```python
from build123d import *

# Parameters (mm, degrees)
ESQUISSE1_W             = 30
ESQUISSE1_H             = 1
ESQUISSE7_R             = 1.7
ENL_V_MAT_EXTRU_1_DEPTH = 33.023428923
ESQUISSE8_R             = 1.6
ENL_V_MAT_EXTRU_2_DEPTH = 32.705677725


with BuildPart() as part:
    # Balayage1: sweep along a path in Esquisse6
    with BuildLine(Plane(origin=(0, 0, 0), x_dir=(0, 0, -1), z_dir=(1, 0, 0))) as balayage1_path:
        Line((0, 0), (20, 0))
        Line((20, 0), (20, -20))
    # Esquisse1 → Balayage1 (sweep)
    with BuildSketch(Plane.XY):
        Rectangle(ESQUISSE1_W, ESQUISSE1_H)
    sweep(path=balayage1_path.line, transition=Transition.RIGHT)

    # Esquisse7 → Enlèv. mat.-Extru.1 (cut, through all)
    with BuildSketch(Plane.XZ.offset(0.5)):
        with Locations(Location((11.49340839, -3, 0), (0, 0, 270))):
            Circle(ESQUISSE7_R)
        with Locations(Location((-10.50659161, -13, 0), (0, 0, 270))):
            Circle(ESQUISSE7_R)
    extrude(amount=-ENL_V_MAT_EXTRU_1_DEPTH, mode=Mode.SUBTRACT)

    # Esquisse8 → Enlèv. mat.-Extru.2 (cut, through all)
    with BuildSketch(Plane.XY.offset(-19.5)):
        with Locations((-10, -9.5)):
            Circle(ESQUISSE8_R)
        with Locations(Location((10, -9.5, 0), (0, 0, 180))):
            Circle(ESQUISSE8_R)
    extrude(amount=-ENL_V_MAT_EXTRU_2_DEPTH, mode=Mode.SUBTRACT)


solid = part.part
```
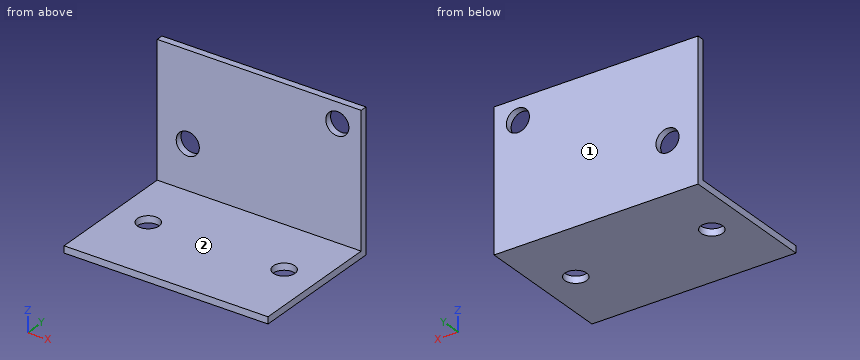
Source: CAD feature listing. Evaluate the final solid. Frame: model axes, mm. Face numbers are marked on the shaded views. A direction names the side the tool comes from. Round coordinates to 2 decimals unless told otherwise and drop trailing zeros. Loops run counter-clockwise (first coordinate to the right, second up) from the corner with the lowest first, then second, coordinate; pieces in that order, holes last. Notation, with made-up numbers: M -23.5,62.25 L 29.5,62.25 A21 cw 29.5,76.25 Z; hole C -33,17 d7. An arc over 180 degrees is marked long. Put each result on its own line as item: value.
(1) First-contact query: pin 1 (10 mm diameter, centred on x = 0, y = -15, fed in from +Z); pin 2 (5 mm diameter, centred on y = -11.5, z = -17.5, fed in from -X); pin 3 (12 mm diameter, centred on y = -9.5, z = -11, fed in from +X); pin 4 (5.5 mm diameter, centred on x = -10.51, z = -13, fed in from -Y). Flat tips, straight axial feed; report the tip coordinate or a pass-through.
Solutions:
pin 1: z = -19.5
pin 2: x = -15
pin 3: through
pin 4: y = -0.5
(2) Section C-C, the plane x = -10. Return loops of the section in (y, z), and give its area (3 significant figures).
Solutions:
outline: M -20,-20.5 L -11.1,-20.5 L -11.1,-19.5 L -20,-19.5 Z; M -7.9,-20.5 L 0.5,-20.5 L 0.5,-14.62 L -0.5,-14.62 L -0.5,-19.5 L -7.9,-19.5 Z; M -0.5,-11.38 L 0.5,-11.38 L 0.5,0 L -0.5,0 Z
area: 33.6 mm²
(3) Section D-D, the plane x = 12.25. Return loops of the section in (y, z).
Solutions:
outline: M -20,-20.5 L 0.5,-20.5 L 0.5,-4.52 L -0.5,-4.52 L -0.5,-19.5 L -20,-19.5 Z; M -0.5,-1.48 L 0.5,-1.48 L 0.5,0 L -0.5,0 Z
(4) Section A-A, the plane z = -13. Return loops of the section in (x, y).
Solutions:
outline: M -15,-0.5 L -12.21,-0.5 L -12.21,0.5 L -15,0.5 Z; M -8.81,-0.5 L 15,-0.5 L 15,0.5 L -8.81,0.5 Z
(5) Section B-B, the plane y = -9.5. Return loops of the section in (x, z).
Solutions:
outline: M -15,-20.5 L -11.6,-20.5 L -11.6,-19.5 L -15,-19.5 Z; M -8.4,-20.5 L 8.4,-20.5 L 8.4,-19.5 L -8.4,-19.5 Z; M 11.6,-20.5 L 15,-20.5 L 15,-19.5 L 11.6,-19.5 Z
(6) Access query for the marked faces 1 and 2. Directions: +Z, -Z, +X, -X, +Y, -Y. A direction counts if a zero-diameter tool reaches every point of the face in a straight line with its end or side. Return the directions, or none.
Solutions:
face 1: +Z, -Z, +X, -X, +Y
face 2: +Z, +X, -X, -Y
(7) Ray query, line 1 (X direction, y = 0, z = -3); line 2 (Y direction, x = -10, z = -20); line 3 (Z direction, x = 0, y = -2.5). Return the intervals inside material, ascending. Write a range as [from, to].
Solutions:
line 1: [-15, 9.79], [13.19, 15]
line 2: [-20, -11.1], [-7.9, 0.5]
line 3: [-20.5, -19.5]
